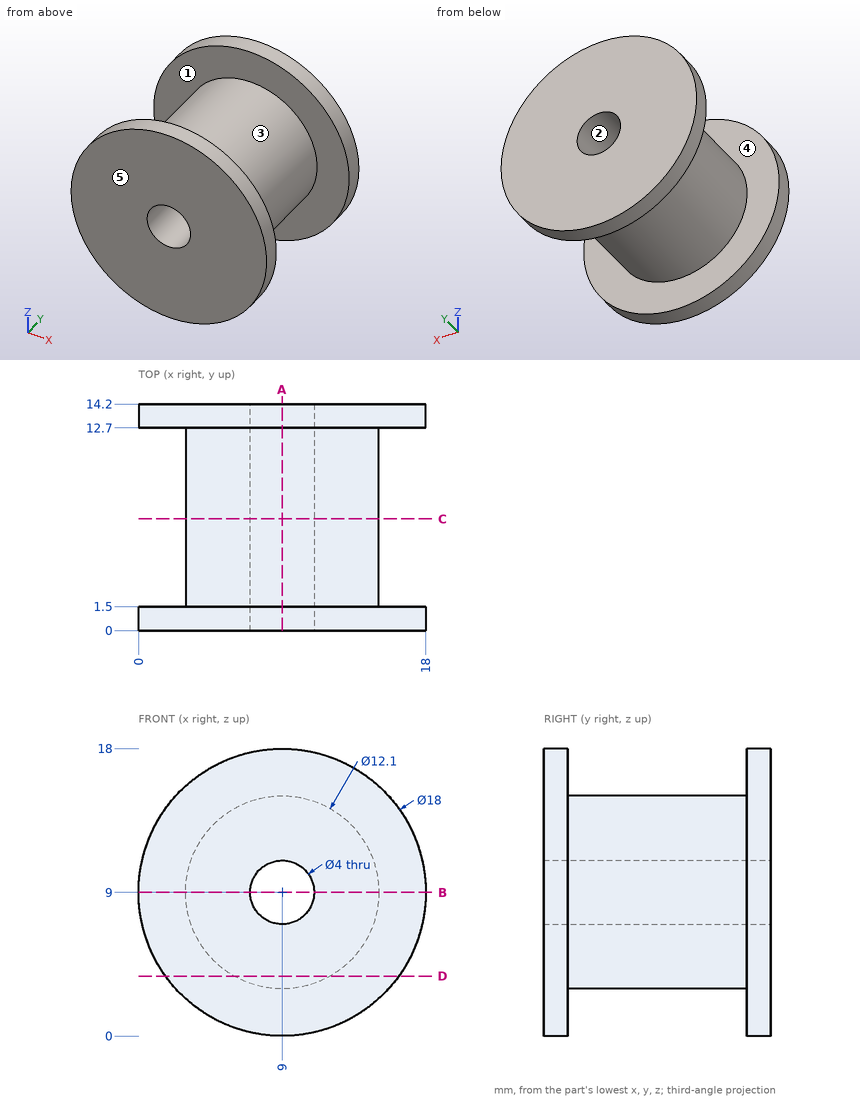
Answer from the drawing. Dimensions are ordinates in mm from the lowest x, y and z of the part. A direction names the side the tool comes from. Give positions to 0.01 mm unless a question says otherwise; leave off trailing zeros. Order: outer loops, then holes, each group sorted by start corner. A loop starts at its lowest first (then second) coordinate and runs counter-clockwise, first axis right, second up. Notation, with made-up numbers: (23, 72.5) -> (34, 72.5) arc R26 ccw to (34, 99.5) -> close; hole circle Ø1 at (1, 63.25). An arc over 180 degrees is marked (long way). One line per item, written item: value. Start each with the question number.
(1) A tool of negligible diameter and unlimited length cuts with its end or side. For the marked faces 4 and 5, from which of +Z, -Z, +X, -X, +Y, -Y can it reach the whole face along a straight path? Write none if from no direction.
(2) The part is cut by section A-A (x = 9). Determine the outline of the cut face in (y, z).
(3) Flat-ended cylindrical pins translate along their axes: P1, Ø3, axis at x = 5.5, y = 3.5, coming from the +Z side; P2, Ø3, axis at x = 2, y = 12.5, coming from the +Z side; P3, Ø1, axis at y = 8.5, z = 8, coming from the -X side. Find the tip coordinate at first contact, or state that the pin passes through.
(4) The part is cut by section D-D (z = 3.75). Determine the outline of the cut face in (x, y).
(5) The part is cut by section C-C (y = 7). Determine the outline of the cut face in (x, z), and give its area (3 significant figures).
(6) Straight lines are drawn through the part: L1, parallel to Y at x = 5.5, z = 16.25; L2, parallel to X at y = 4, z = 9. For each, find the intervals that lie inside material, in ascending order.
(7) For a pull along Z with two mould halves and no side action, classify the marked faces 1, 2 and 3 as released by +Z, released by -Z, zero draft, split by the parting line, or undercut.
(8) The part is cut by section B-B (z = 9). Determine the outline of the cut face in (x, y).
Taken from the geometry:
1. face 4: none
1. face 5: +Z, -Z, +X, -X, -Y
2. outline: (0, 0) -> (1.5, 0) -> (1.5, 2.95) -> (12.7, 2.95) -> (12.7, 0) -> (14.2, 0) -> (14.2, 7) -> (0, 7) -> close; (0, 11) -> (14.2, 11) -> (14.2, 18) -> (12.7, 18) -> (12.7, 15.05) -> (1.5, 15.05) -> (1.5, 18) -> (0, 18) -> close
3. P1: z = 14.71
3. P2: z = 16.11
3. P3: x = 2.97
4. outline: (1.69, 0) -> (16.31, 0) -> (16.31, 1.5) -> (12.01, 1.5) -> (12.01, 12.7) -> (16.31, 12.7) -> (16.31, 14.2) -> (1.69, 14.2) -> (1.69, 12.7) -> (5.99, 12.7) -> (5.99, 1.5) -> (1.69, 1.5) -> close
5. outline: circle Ø12.1 at (9, 9); hole circle Ø4 at (9, 9)
5. area: 102 mm^2
6. L1: 0 to 1.5, 12.7 to 14.2
6. L2: 2.95 to 7, 11 to 15.05
7. face 1: zero draft
7. face 2: undercut
7. face 3: split by the parting line
8. outline: (0, 0) -> (7, 0) -> (7, 14.2) -> (0, 14.2) -> (0, 12.7) -> (2.95, 12.7) -> (2.95, 1.5) -> (0, 1.5) -> close; (11, 0) -> (18, 0) -> (18, 1.5) -> (15.05, 1.5) -> (15.05, 12.7) -> (18, 12.7) -> (18, 14.2) -> (11, 14.2) -> close
